Could you check a few things on this model? Use its own coordinates, in mm. Face numbers are marked on the shaded views. A direction names the side the tool comes from. Give positions to 0.01 mm unless a question says otherwise; leave off trailing zeros. Loops run counter-clockwise (first coordinate to the right, second up) from the corner with the lowest first, then second, coordinate; pieces in that order, holes last. Notation, with made-up numbers: M 36.5,-33 L 51.5,-33 A20 ccw 51.5,-13 Z; hole C 80.5,-4.75 d10. An arc over 180 degrees is marked long. Use CSV: the item, a comma, the result in double quotes.
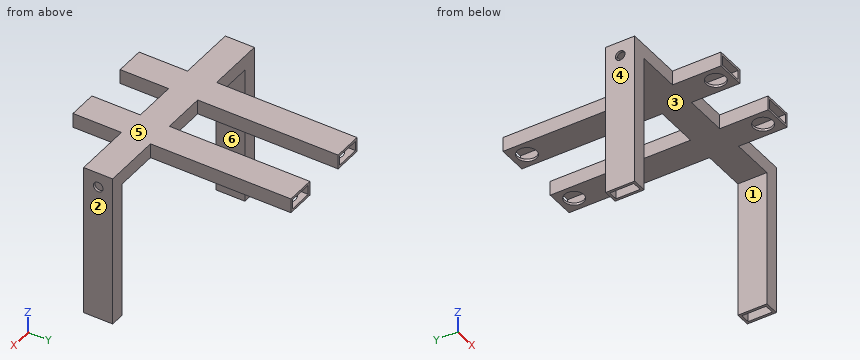
Autodesk Inventor part; units mm, degrees
ref_plane "Work Plane1" through (0, 0, -190.5) normal (0, 0, 1) x (1, 0, 0)
ref_plane "XZ Plane" through (0, 0, 0) normal (0, 1, 0) x (-1, 0, 0)
sketch "Sketch1" plane through (0, 0, 0) normal (0, 1, 0) x (-1, 0, 0)
  line L0 (0, 0) -> (133.35, 0)
  line L1 (133.35, 0) -> (133.35, -190.5)
  line L2 (0, 0) -> (0, -190.5) construction
  line L3 (0, 0) -> (-133.35, 0)
  line L4 (-133.35, 0) -> (-133.35, -190.5)
  dimension "d0" = 133.35
  dimension "d1" = 190.5
  dimension "d2" = 190.5
ref_plane "Work Plane1" through (0, 0, -190.5) normal (0, 0, 1) x (1, 0, 0)
sketch "Sketch3" plane through (0, 0, -190.5) normal (0, 0, 1) x (1, 0, 0)
  line L0 (142.875, -19.05) -> (123.825, -19.05)
  line L1 (123.825, -19.05) -> (123.825, 19.05)
  line L2 (123.825, 19.05) -> (142.875, 19.05)
  line L3 (142.875, 19.05) -> (142.875, -19.05)
  line L4 (142.875, -19.05) -> (123.825, 19.05) construction
  line L5 (123.825, -19.05) -> (142.875, 19.05) construction
  line L6 (139.7, -15.875) -> (127, -15.875)
  line L7 (127, -15.875) -> (127, 15.875)
  line L8 (127, 15.875) -> (139.7, 15.875)
  line L9 (139.7, 15.875) -> (139.7, -15.875)
  line L10 (139.7, -15.875) -> (127, 15.875) construction
  line L11 (127, -15.875) -> (139.7, 15.875) construction
  point P0 (0, 0)
  point P1 (133.35, 0)
  dimension "d4" = 38.1
  dimension "d5" = 19.05
  dimension "d6" = 133.35
  dimension "d7" = 3.175
  dimension "d8" = 3.175
sweep "Sweep1" add profiles "Sketch3" path "Sketch1"
sketch "Sketch4" plane through (123.825, 19.05, -190.5) normal (0, 1, 0) x (1, 0, 0)
  line L0 (-190.5, -200.025) -> (-152.4, -200.025)
  line L1 (-152.4, -200.025) -> (-152.4, -180.975)
  line L2 (-152.4, -180.975) -> (-190.5, -180.975)
  line L3 (-190.5, -180.975) -> (-190.5, -200.025)
  line L4 (-190.5, -200.025) -> (-152.4, -180.975) construction
  line L5 (-152.4, -200.025) -> (-190.5, -180.975) construction
  line L6 (-266.7, -200.025) -> (-266.7, 0)
  line L7 (-187.325, -196.85) -> (-155.575, -196.85)
  line L8 (-155.575, -196.85) -> (-155.575, -184.15)
  line L9 (-155.575, -184.15) -> (-187.325, -184.15)
  line L10 (-187.325, -184.15) -> (-187.325, -196.85)
  line L11 (-187.325, -196.85) -> (-155.575, -184.15) construction
  line L12 (-155.575, -196.85) -> (-187.325, -184.15) construction
  line L13 (3.175, -184.15) -> (-250.825, -184.15)
  point P0 (-123.825, -190.5)
  point P1 (-171.45, -190.5)
  dimension "d11" = 95.25
  dimension "d12" = 19.05
  dimension "d13" = 38.1
  dimension "d14" = 3.175
  dimension "d15" = 3.175
extrude "Extrusion1" add sketch "Sketch4" along normal blind 184.15 contours L3 L13 L10 L7 L8 L1 L0 | L3 L2 L1 L13 L9
sketch "Sketch5" plane through (123.825, -19.05, -190.5) normal (0, -1, 0) x (1, 0, 0)
  line L0 (-190.5, 180.975) -> (-152.4, 180.975)
  line L1 (-152.4, 180.975) -> (-152.4, 200.025)
  line L2 (-152.4, 200.025) -> (-190.5, 200.025)
  line L3 (-190.5, 200.025) -> (-190.5, 180.975)
  line L4 (-190.5, 180.975) -> (-152.4, 200.025) construction
  line L5 (-152.4, 180.975) -> (-190.5, 200.025) construction
  line L6 (-266.7, 200.025) -> (-266.7, 0)
  line L7 (-187.325, 184.15) -> (-155.575, 184.15)
  line L8 (-155.575, 184.15) -> (-155.575, 196.85)
  line L9 (-155.575, 196.85) -> (-187.325, 196.85)
  line L10 (-187.325, 196.85) -> (-187.325, 184.15)
  line L11 (-187.325, 184.15) -> (-155.575, 196.85) construction
  line L12 (-155.575, 184.15) -> (-187.325, 196.85) construction
  point P0 (-123.825, 190.5)
  point P1 (-171.45, 190.5)
  dimension "d18" = 95.25
  dimension "d19" = 19.05
  dimension "d20" = 38.1
  dimension "d21" = 3.175
  dimension "d22" = 3.175
extrude "Extrusion2" add sketch "Sketch5" along normal blind 63.5
mirror "Mirror1" about plane through (0, 0, 0) normal (1, 0, 0) of "Extrusion1", "Extrusion2"
sketch "Sketch6" plane through (142.875, -19.05, -190.5) normal (1, 0, 0) x (0, 0, -1)
  line L0 (-200.025, 0) -> (-200.025, 38.1)
  point P0 (-190.5, 19.05)
  point P1 (-180.975, 19.05)
  dimension "d25" = 19.05
hole "Hole1" at (142.875, 0, -9.525) direction (-1, 0, 0) diameter 12.7 depth 3.175 tip angle 118
sketch "Sketch7" plane through (-66.675, 19.05, -9.525) normal (0, 0, -1) x (-1, 0, 0)
  line L0 (-38.1, 184.15) -> (0, 184.15) construction
  line L1 (-19.05, 184.15) -> (-19.05, -101.6) construction
  line L2 (-34.925, -101.6) -> (-3.175, -101.6) construction
  line L3 (-95.25, 184.15) -> (-133.35, 184.15) construction
  line L4 (-114.3, 184.15) -> (-114.3, -101.6) construction
  line L5 (-133.35, -101.6) -> (-95.25, -101.6) construction
  point P0 (-66.675, -19.05)
  point P1 (-19.05, 165.1)
  point P2 (-19.05, -82.55)
  point P3 (-114.3, -82.55)
  point P4 (-114.3, 165.1)
  dimension "d33" = 19.05
  dimension "d34" = 19.05
  dimension "d35" = 19.05
  dimension "d36" = 19.05
hole "Hole2" at (-47.625, 184.15, -9.525) at (-47.625, -63.5, -9.525) at (47.625, -63.5, -9.525) at (47.625, 184.15, -9.525) direction (0, 0, 1) diameter 25.4 depth 3.175 tip angle 118
mirror "Mirror2" about plane through (0, 0, 0) normal (1, 0, 0) of "Hole1"
equation "\"d0\" = 0.5 * width"
equation "\"d1\" = length"
equation "\"d2\" = length"
equation "\"d4\" = tubingLength"
equation "\"d5\" = tubingWidth"
equation "\"d7\" = tubeingWallWidth"
equation "\"d8\" = tubeingWallWidth"
equation "\"d12\" = tubingWidth"
equation "\"d13\" = tubingLength"
equation "\"d14\" = tubeingWallWidth"
equation "\"d15\" = tubeingWallWidth"
equation "\"d19\" = tubingWidth"
equation "\"d20\" = tubingLength"
equation "\"d21\" = tubeingWallWidth"
equation "\"d22\" = tubeingWallWidth"
equation "\"width\" = 266.7"
equation "\"length\" = 190.5"
equation "\"tubingWidth\" = 19.05"
equation "\"tubingLength\" = 38.1"
equation "\"tubeingWallWidth\" = 3.175"
equation "\"d3\" = -length"
properties part number "Shooter"
1. I want a section at B-B, the plane z = -173.5. List the corners of the cut face in (x, y) for me (3 decimals).
Outcome:
outline,"M -142.875,-19.05 L -123.825,-19.05 L -123.825,19.05 L -142.875,19.05 Z; M 123.825,-19.05 L 142.875,-19.05 L 142.875,19.05 L 123.825,19.05 Z; hole M -139.7,-15.875 L -127,-15.875 L -127,15.875 L -139.7,15.875 Z; hole M 127,-15.875 L 139.7,-15.875 L 139.7,15.875 L 127,15.875 Z"
2. I'm going to push flat-ended pins straight in: pin 1 Ø5.5 at (y, z) = (80.5, -3.5) entering from +X (3 decimals); pin 2 Ø16 at (x, y) = (4, -1.5) entering from -Z (3 decimals); pin 3 Ø6.5 at (x, z) = (48.5, 3) entering from +Y; pin 4 Ø14.5 at (y, z) = (0, -9.525) entering from +X (3 decimals). Where does each tip first touch, or does it pass through?
Outcome:
pin 1,"x = 66.675"
pin 2,"z = -9.525"
pin 3,"y = 19.05"
pin 4,"x = 142.875"
3. I want a section at C-C, the plane x = 51.5. List the corners of the cut face in (y, z) for me (3 decimals).
Outcome:
outline,"M -82.55,-9.525 L -75.594,-9.525 L -75.594,-6.35 L -82.55,-6.35 Z; M -82.55,6.35 L -19.05,6.35 L -19.05,-6.35 L -51.406,-6.35 L -51.406,-9.525 L 172.056,-9.525 L 172.056,-6.35 L 19.05,-6.35 L 19.05,6.35 L 203.2,6.35 L 203.2,9.525 L -82.55,9.525 Z; M 196.244,-9.525 L 203.2,-9.525 L 203.2,-6.35 L 196.244,-6.35 Z; hole M -15.875,-6.35 L 15.875,-6.35 L 15.875,6.35 L -15.875,6.35 Z"
4. If we mould it in two halves opening along X, with no side actions, what happens to the marked faces 1, 2, 3 and 4? For each: +X half, -X half, draft (parallel to the pull), parting line (faces both ways), or undercut.
Outcome:
face 1,"undercut"
face 2,"+X half"
face 3,"undercut"
face 4,"-X half"
5. Which directions (+Z, -Z, +X, -X, +Y, -Y) give clear straight access to the entire face, cutting with the end or side of a thin tool? Please do the marked faces 5 and 6.
Outcome:
face 5,"+Z, +X, -X, +Y, -Y"
face 6,"-Z, +Y, -Y"
6. Please list where these lines run through material, in increasing order: line 1 (X direction, y = -8.5, z = -165) (3 decimals); line 2 (X direction, y = -30, z = -0.5) (3 decimals); line 3 (Z direction, x = -65.5, y = 11) (3 decimals).
Outcome:
line 1,"-142.875 to -139.7, -127 to -123.825, 123.825 to 127, 139.7 to 142.875"
line 2,"-66.675 to -63.5, -31.75 to -28.575, 28.575 to 31.75, 63.5 to 66.675"
line 3,"-9.525 to -6.35, 6.35 to 9.525"
7. I want a section at A-A, the plane y = 85.5. List the corners of the cut face in (x, z) for me (3 decimals), then the cut area to 3 significant figures.
Outcome:
outline,"M -66.675,-9.525 L -28.575,-9.525 L -28.575,9.525 L -66.675,9.525 Z; M 28.575,-9.525 L 66.675,-9.525 L 66.675,9.525 L 28.575,9.525 Z; hole M -63.5,-6.35 L -31.75,-6.35 L -31.75,6.35 L -63.5,6.35 Z; hole M 31.75,-6.35 L 63.5,-6.35 L 63.5,6.35 L 31.75,6.35 Z"
area,"645 mm2"
8. I want a section at D-D, the plane y = 0. List the corners of the cut face in (x, z) for me (3 decimals), then the cut area to 3 significant figures.
Outcome:
outline,"M -142.875,-190.5 L -139.7,-190.5 L -139.7,-15.875 L -142.875,-15.875 Z; M -142.875,-3.175 L -139.7,-3.175 L -139.7,6.35 L 139.7,6.35 L 139.7,-3.175 L 142.875,-3.175 L 142.875,9.525 L -142.875,9.525 Z; M -127,-190.5 L -123.825,-190.5 L -123.825,-9.525 L 123.825,-9.525 L 123.825,-190.5 L 127,-190.5 L 127,-6.35 L -127,-6.35 Z; M 139.7,-190.5 L 142.875,-190.5 L 142.875,-15.875 L 139.7,-15.875 Z"
area,"4,030 mm2"
